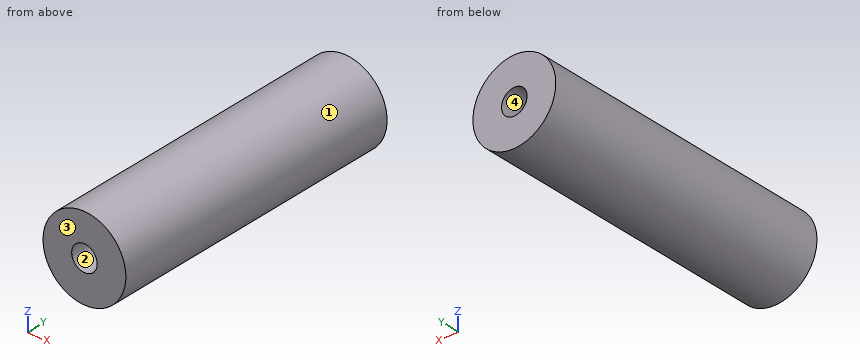
Autodesk Inventor part; units mm, degrees
ref_plane "Work Plane1" through (0, 14.55, 0) normal (0, 1, 0) x (1, 0, 0)
ref_plane "YZ Plane" through (0, 0, 0) normal (1, 0, 0) x (0, 1, 0)
ref_plane "XZ Plane" through (0, 0, 0) normal (0, 1, 0) x (-1, 0, 0)
sketch "Sketch1" plane through (0, 0, 0) normal (0, 1, 0) x (-1, 0, 0)
  circle A0 centre (0, 0) radius 4
  dimension "d0" = 8
extrude "Extrusion1" add sketch "Sketch1" along normal blind 29.1
sketch "Sketch2" plane through (0, 29.1, 0) normal (0, 1, 0) x (1, 0, 0)
  point P0 (0, 0)
  point P1 (0, 0)
hole "Hole1" at (0, 29.1, 0) direction (0, -1, 0) diameter 2.459 depth 8.8 tip angle 118
ref_plane "Work Plane1" through (0, 14.55, 0) normal (0, 1, 0) x (1, 0, 0)
mirror "Mirror1" about plane through (0, 14.55, 0) normal (0, 1, 0) of "Hole1"
properties part number "rod mount motor"
Geometry check sheet. Reference: the model listing, model coordinates, mm. Face numbers are marked on the shaded views. Coordinates: 2 decimals unless noted, no trailing zeros. Loops run counter-clockwise (first coordinate to the right, second up) from the corner with the lowest first, then second, coordinate; pieces in that order, holes last.
Item 1: Release check for a two-part mould opening along Z. For the marked faces 1, 2, 3 and 4 record: released by +Z, released by -Z, zero draft, split by the parting line, or undercut.
Item 2: Thickness scan on line 1 (Z direction, x = 0, y = 22.25); line 2 (X direction, y = 20.75, z = -1); line 3 (Z direction, x = -0.75, y = 23.25). Record the ranges inside material, lowest first.
Item 3: Go/stop test with a flat-tipped pin: pin 1 Ø2 at (y, z) = (14, -3) entering from +X. Record where the tip stops, or that it passes through.
Item 4: Sectioned sample at B-B, the plane y = 7.5. Record the boundary of the cut face in (x, z), then the cut area to 3 significant figures.
Item 5: Sectioned sample at C-C, the plane x = 1.75. Record the boundary of the cut face in (y, z).
Item 6: Sectioned sample at A-A, the plane y = 19. Record the boundary of the cut face in (x, z).
Item 7: Sectioned sample at D-D, the plane z = -1.75. Record the boundary of the cut face in (x, y).
Check result:
1. face 1: split by the parting line
1. face 2: undercut
1. face 3: zero draft
1. face 4: undercut
2. line 1: z = -4 to -1.23, 1.23 to 4
2. line 2: x = -3.87 to -0.72, 0.72 to 3.87
2. line 3: z = -3.93 to -0.97, 0.97 to 3.93
3. pin 1: stops at x = 3.46
4. outline: circle Ø8 at (0, 0); hole circle Ø2.46 at (0, 0)
4. area: 45.5 mm2
5. outline: (0, -3.6) - (29.1, -3.6) - (29.1, 3.6) - (0, 3.6) - close
6. outline: circle Ø8 at (0, 0)
7. outline: (-3.6, 0) - (3.6, 0) - (3.6, 29.1) - (-3.6, 29.1) - close
